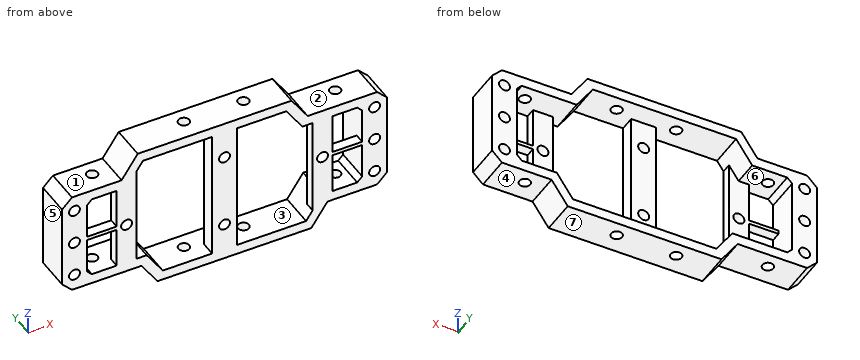
from build123d import *

# Parameters (mm, degrees)
BOSS_EXTRUDE1_DEPTH = 14
CUT_EXTRUDE1_REACH  = 16
SKETCH2_R           = 2.2
SKETCH5_R           = 2.2
CUT_EXTRUDE2_DEPTH  = 62
BOSS_EXTRUDE2_REACH = 59
SKETCH6_W           = 10
SKETCH6_H           = 6
SKETCH7_W           = 12
SKETCH7_H           = 1.5
SKETCH7_R           = 2.2
BOSS_EXTRUDE3_DEPTH = 4
CUT_EXTRUDE3_REACH  = 16
SKETCH8_R           = 2.2
CHAMFER1_SIZE       = 4
CHAMFER2_SIZE       = 2


with BuildPart() as part:
    # Sketch1 → Boss-Extrude1 (new body)
    with BuildSketch(Plane(origin=(0, 0, 0), x_dir=(1, 0, 0), z_dir=(0, 1, 0))):
        Polygon((-104.176003517, -21), (-104.176003517, 21), (-72.176003517, 21), (-65.676003517, 30.5), (-3.676003517, 30.5), (2.823996483, 21), (26.823996483, 21), (26.823996483, -21), (-5.176003517, -21), (-11.676003517, -30.5), (-73.676003517, -30.5), (-80.176003517, -21), align=None)
        Polygon((-94.176003517, -17), (-94.176003517, 17), (-70.066165861, 17), (-63.566165861, 26.5), (-5.785841173, 26.5), (0.714158827, 17), (16.823996483, 17), (16.823996483, -17), (-7.285841173, -17), (-13.785841173, -26.5), (-71.566165861, -26.5), (-78.066165861, -17), align=None, mode=Mode.SUBTRACT)
    extrude(amount=BOSS_EXTRUDE1_DEPTH)

    # Sketch2 → Cut-Extrude1 (cut, up to next)
    with BuildSketch(Plane(origin=(0, 0, 0), x_dir=(-1, 0, 0), z_dir=(0, -1, 0)), mode=Mode.PRIVATE) as cut_extrude1_sk1:
        with Locations(Location((99.176003517, 14.5, 0), (0, 0, 90))):  # turned: the seam where the file's is
            Circle(SKETCH2_R)
    cut_extrude1_tool1 = extrude(cut_extrude1_sk1.sketch, amount=-CUT_EXTRUDE1_REACH, mode=Mode.PRIVATE) & part.part
    add(cut_extrude1_tool1.solids().sort_by_distance((-99.176004, 0, -14.5))[0], mode=Mode.SUBTRACT)
    # Sketch2 → Cut-Extrude1 (cut, up to next)
    with BuildSketch(Plane(origin=(0, 0, 0), x_dir=(-1, 0, 0), z_dir=(0, -1, 0)), mode=Mode.PRIVATE) as cut_extrude1_sk2:
        with Locations(Location((99.176003517, 0, 0), (0, 0, 90))):  # turned: the seam where the file's is
            Circle(SKETCH2_R)
    cut_extrude1_tool2 = extrude(cut_extrude1_sk2.sketch, amount=-CUT_EXTRUDE1_REACH, mode=Mode.PRIVATE) & part.part
    add(cut_extrude1_tool2.solids().sort_by_distance((-99.176004, 0, 0))[0], mode=Mode.SUBTRACT)
    # Sketch2 → Cut-Extrude1 (cut, up to next)
    with BuildSketch(Plane(origin=(0, 0, 0), x_dir=(-1, 0, 0), z_dir=(0, -1, 0)), mode=Mode.PRIVATE) as cut_extrude1_sk3:
        with Locations(Location((99.176003517, -14.5, 0), (0, 0, 90))):  # turned: the seam where the file's is
            Circle(SKETCH2_R)
    cut_extrude1_tool3 = extrude(cut_extrude1_sk3.sketch, amount=-CUT_EXTRUDE1_REACH, mode=Mode.PRIVATE) & part.part
    add(cut_extrude1_tool3.solids().sort_by_distance((-99.176004, 0, 14.5))[0], mode=Mode.SUBTRACT)
    # Sketch2 → Cut-Extrude1 (cut, up to next)
    with BuildSketch(Plane(origin=(0, 0, 0), x_dir=(-1, 0, 0), z_dir=(0, -1, 0)), mode=Mode.PRIVATE) as cut_extrude1_sk4:
        with Locations(Location((-21.823996483, -14.5, 0), (0, 0, 90))):  # turned: the seam where the file's is
            Circle(SKETCH2_R)
    cut_extrude1_tool4 = extrude(cut_extrude1_sk4.sketch, amount=-CUT_EXTRUDE1_REACH, mode=Mode.PRIVATE) & part.part
    add(cut_extrude1_tool4.solids().sort_by_distance((21.823996, 0, 14.5))[0], mode=Mode.SUBTRACT)
    # Sketch2 → Cut-Extrude1 (cut, up to next)
    with BuildSketch(Plane(origin=(0, 0, 0), x_dir=(-1, 0, 0), z_dir=(0, -1, 0)), mode=Mode.PRIVATE) as cut_extrude1_sk5:
        with Locations(Location((-21.823996483, 0, 0), (0, 0, 90))):  # turned: the seam where the file's is
            Circle(SKETCH2_R)
    cut_extrude1_tool5 = extrude(cut_extrude1_sk5.sketch, amount=-CUT_EXTRUDE1_REACH, mode=Mode.PRIVATE) & part.part
    add(cut_extrude1_tool5.solids().sort_by_distance((21.823996, 0, 0))[0], mode=Mode.SUBTRACT)
    # Sketch2 → Cut-Extrude1 (cut, up to next)
    with BuildSketch(Plane(origin=(0, 0, 0), x_dir=(-1, 0, 0), z_dir=(0, -1, 0)), mode=Mode.PRIVATE) as cut_extrude1_sk6:
        with Locations(Location((-21.823996483, 14.5, 0), (0, 0, 90))):  # turned: the seam where the file's is
            Circle(SKETCH2_R)
    cut_extrude1_tool6 = extrude(cut_extrude1_sk6.sketch, amount=-CUT_EXTRUDE1_REACH, mode=Mode.PRIVATE) & part.part
    add(cut_extrude1_tool6.solids().sort_by_distance((21.823996, 0, -14.5))[0], mode=Mode.SUBTRACT)

    # Sketch5 → Cut-Extrude2 (cut, through all)
    with BuildSketch(Plane(origin=(0, 0, -30.5), x_dir=(-1, 0, 0), z_dir=(0, 0, -1))):
        with Locations((50.676003517, 8)):
            Circle(SKETCH5_R)
        with Locations((26.676003517, 8)):
            Circle(SKETCH5_R)
        with Locations(Location((87.676003517, 8, 0), (0, 0, 180))):  # turned: the seam where the file's is
            Circle(SKETCH5_R)
        with Locations(Location((-10.323996483, 8, 0), (0, 0, 180))):  # turned: the seam where the file's is
            Circle(SKETCH5_R)
    extrude(amount=-CUT_EXTRUDE2_DEPTH, mode=Mode.SUBTRACT)

    # Sketch6 → Boss-Extrude2 (add, up to next)
    with BuildSketch(Plane(origin=(0, 0, 26.5), x_dir=(-1, 0, 0), z_dir=(0, 0, -1)), mode=Mode.PRIVATE) as boss_extrude2_sk1:
        with Locations((38.676003517, 3)):
            Rectangle(SKETCH6_W, SKETCH6_H)
    boss_extrude2_tool1 = extrude(boss_extrude2_sk1.sketch, amount=BOSS_EXTRUDE2_REACH, mode=Mode.PRIVATE) - part.part
    add(boss_extrude2_tool1.solids().sort_by_distance((-38.676004, 3, 26.5))[0])

    # Sketch7 → Boss-Extrude3 (add)
    with BuildSketch(Plane.XZ):
        with Locations((-88.176003517, 0)):
            Rectangle(SKETCH7_W, SKETCH7_H)
        Polygon((-78.066165861, 17), (-82.176003517, 17), (-82.176003517, 0.75), (-82.176003517, -0.75), (-82.176003517, -17), (-74.176003517, -17), (-74.176003517, 22.685621887), align=None)
        with Locations(Location((-78.176003517, 0, 0), (0, 0, 270))):  # turned: the seam where the file's is
            Circle(SKETCH7_R, mode=Mode.SUBTRACT)
        Polygon((4.823996483, 0.75), (4.823996483, 17), (-3.176003517, 17), (-3.176003517, -22.685621887), (0.714158827, -17), (4.823996483, -17), (4.823996483, -0.75), align=None)
        with Locations(Location((0.823996483, 0, 0), (0, 0, 270))):  # turned: the seam where the file's is
            Circle(SKETCH7_R, mode=Mode.SUBTRACT)
        with Locations((10.823996483, 0)):
            Rectangle(SKETCH7_W, SKETCH7_H)
    extrude(amount=-BOSS_EXTRUDE3_DEPTH)

    # Sketch8 → Cut-Extrude3 (cut, up to next)
    with BuildSketch(Plane(origin=(0, 0, 0), x_dir=(-1, 0, 0), z_dir=(0, -1, 0)), mode=Mode.PRIVATE) as cut_extrude3_sk1:
        with Locations(Location((38.676003517, -15.25, 0), (0, 0, 90))):  # turned: the seam where the file's is
            Circle(SKETCH8_R)
    cut_extrude3_tool1 = extrude(cut_extrude3_sk1.sketch, amount=-CUT_EXTRUDE3_REACH, mode=Mode.PRIVATE) & part.part
    add(cut_extrude3_tool1.solids().sort_by_distance((-38.676004, 0, 15.25))[0], mode=Mode.SUBTRACT)
    # Sketch8 → Cut-Extrude3 (cut, up to next)
    with BuildSketch(Plane(origin=(0, 0, 0), x_dir=(-1, 0, 0), z_dir=(0, -1, 0)), mode=Mode.PRIVATE) as cut_extrude3_sk2:
        with Locations(Location((38.676003517, 15.25, 0), (0, 0, 90))):  # turned: the seam where the file's is
            Circle(SKETCH8_R)
    cut_extrude3_tool2 = extrude(cut_extrude3_sk2.sketch, amount=-CUT_EXTRUDE3_REACH, mode=Mode.PRIVATE) & part.part
    add(cut_extrude3_tool2.solids().sort_by_distance((-38.676004, 0, -15.25))[0], mode=Mode.SUBTRACT)

    # Chamfer1
    chamfer1_edges = [part.edges().sort_by_distance(p)[0] for p in [
        (-104.176003517, 7, 21),
        (-104.176003517, 7, -21),
        (26.823996483, 7, -21),
        (26.823996483, 7, 21),
    ]]
    chamfer(chamfer1_edges, length=CHAMFER1_SIZE)

    # Chamfer2
    chamfer2_edges = [part.edges().sort_by_distance(p)[0] for p in [
        (-94.176003517, 7, 17),
        (16.823996483, 7, 17),
        (16.823996483, 7, -17),
        (-94.176003517, 7, -17),
    ]]
    chamfer(chamfer2_edges, length=CHAMFER2_SIZE)


solid = part.part
Can you work these out from the model? Positions are in its coordinate system, mm. Face numbers are marked on the shaded views. A direction names the side the tool comes from. Coordinates: 2 decimals unless noted, no trailing zeros. Write each loop counter-clockwise with the first axis right and the second up, starting at its lowest first coordinate (ties: lowest second). Pieces come first, ordered by that corner, then holes. Notation, with made-up numbers: (18.5, 52) -> (62.5, 52) arc R15 ccw to (62.5, 58) -> close; hole circle Ø2 at (-25.75, 87.25). An arc over 180 degrees is marked (long way). Answer as CSV lines item,"result".
1) If I drill on line 1 (X direction, y = 8.5, z = 14.5); line 2 (Z direction, x = -24, y = 9.5); line 3 (X direction, y = 7.25, z = 2), over which ranges is the centre line in solid material (lowest first)? Write a range as from..to.
Check result:
line 1,"-104.18..-101.38, -96.98..-94.18, 16.82..19.62, 24.02..26.82"
line 2,"-30.5..-26.5, 26.5..30.5"
line 3,"-104.18..-100.09, -98.26..-94.18, 16.82..20.91, 22.74..26.82"
2) On a 3-axis mill with a long thin cutter (end or side, diameter ignored), from which of +Z, -Z, +X, -X, +Y, -Y can I reach the whole of each face in a straight line? I mean the marked faces 1, 2, 3 and 4. Say none if no direction works.
Check result:
face 1,"+Z, -X, +Y, -Y"
face 2,"+Z, +X, +Y, -Y"
face 3,"+Y"
face 4,"-Z, +X, +Y, -Y"
3) If we section it at C-C on y = 8: Count the separate pieces of the cut face and the enclosed holes in it, then the cut area to 3 significant figures.
Check result:
separate pieces,"8"
enclosed holes,"6"
area,"1,550 mm²"
4) If we section it at B-B on z = 9.5: Please give me the cut outline in (x, y), then the cut area to 3 significant figures.
Check result:
outline,"(-104.18, 0) -> (-94.18, 0) -> (-94.18, 14) -> (-104.18, 14) -> close; (-82.18, 0) -> (-74.18, 0) -> (-74.18, 4) -> (-82.18, 4) -> close; (-43.68, 0) -> (-33.68, 0) -> (-33.68, 6) -> (-43.68, 6) -> close; (-3.18, 0) -> (4.82, 0) -> (4.82, 4) -> (-3.18, 4) -> close; (16.82, 0) -> (26.82, 0) -> (26.82, 14) -> (16.82, 14) -> close"
area,"404 mm²"
5) If we section it at D-D on x = -9: Please give me the cut outline in (y, z).
Check result:
outline,"(0, -30.5) -> (14, -30.5) -> (14, -26.5) -> (0, -26.5) -> close; (0, 19.51) -> (14, 19.51) -> (14, 26.59) -> (0, 26.59) -> close"
6) If we mould it in two halves opening along X, with no side actions, what happens to the marked faces 5, 6 and 7? For each: +X half, -X half, draft (parallel to the pull), parting line (faces both ways), or undercut.
Check result:
face 5,"-X half"
face 6,"undercut"
face 7,"draft"
7) Will these pins go through, and if not, where does the flat tip stop? P1, Ø2.5, axis at x = 0.82, z = 0, coming from the +Y side; P2, Ø7, axis at x = -87.68, y = 8, coming from the -Z side; P3, Ø5, axis at x = 3.5, y = 11, coming from the +Z side.
Check result:
P1,"through"
P2,"z = -21"
P3,"z = 21"
8) If we section it at A-A on x = -47: Please give me the cut outline in (y, z).
Check result:
outline,"(0, -30.5) -> (14, -30.5) -> (14, -26.5) -> (0, -26.5) -> close; (0, 26.5) -> (14, 26.5) -> (14, 30.5) -> (0, 30.5) -> close"
